For this review, take the finished solid that the model builds, in its own axes (mm). A direction names the side the tool comes from. Coordinates: 2 decimals unless noted, no trailing zeros. Write each loop counter-clockwise with the first axis right and the second up, starting at its lowest first coordinate (ties: lowest second). Pieces come first, ordered by that corner, then holes.
1) For faces 1 (the face through (6.583, 24.324, -1.479)), 2 (the face through (4.31, 17.88, -1.48)), list the 3-axis set-ups (+Z, -Z, +X, -X, +Y, -Y) from which the entire face can be reached by the end or side of a thin tool; tool diameter is ignored.
2) We need section C-C on y = -2.5. Write out the cut boundary in (x, z).
3) Insertion check: P1, Ø1, axis at y = 1, z = -1, coming from the +X side; P2, Ø1.5, axis at y = 2, z = -0.5, coming from the +X side; P3, Ø1.5, axis at x = 1, z = -1, coming from the -Y side. Each pin has a flat end and moves straight along its axis. Give the tip position at first contact, or say it passes through.
4) To check wall thickness, follow line 1 along X through (y, z) = (-4, -2.8); line 2 along Y through (x, z) = (-3.5, -1.55); line 3 along X through (y, z) = (-6, -0.1). State the ranges of each line that lie inside material, in increasing order.
5) Mouldability with a two-part tool opening along X and no side actions: class faces 3 (the face through (-4.88, -8.31, -1.48)), 4 (the face through (9.96, 10.462, -1.479)), 5 (the face through (-4.81, 5.69, -1.48)), 6 (the face through (0, 1, -3)) as pulls with the +X half, pulls with the -X half, needs draft (parallel to the pull), parting line crosses it, or undercut.
6) We need section B-B on z = -1.4. Write out the cut boundary in (x, y).
7) We need section A-A on y = 14. Write out the cut boundary in (x, z), then the cut area to 3 significant figures.
8) We need section D-D on y = -11. Write out the cut boundary in (x, z), then the cut area to 3 significant figures.
from build123d import *

# Parameters (mm, degrees)
F1_DEPTH = 3


with BuildPart() as f1:
    # F0 (on Top) → F1 (new body)
    with BuildSketch(Plane.XY):
        with BuildLine():
            Line((3.145587, 13.081894), (-1.617252, 14.912562))
            ThreePointArc((-1.617252, 14.912562), (-5.38163, -14.001359), (11.189027, 9.990279))
            Line((11.189027, 9.990279), (8.696999, 10.948126))
            ThreePointArc((8.696999, 10.948126), (10.035784, 16.738453), (9.370891, 22.644226))
            ThreePointArc((9.370891, 22.644226), (6.534897, 24.324435), (3.698903, 22.644226))
            ThreePointArc((3.698903, 22.644226), (4.30714, 17.811856), (3.145587, 13.081894))
        make_face()
        with BuildLine():
            ThreePointArc((5.58474, -8.803174), (-6.250082, -12.977674), (-8.510819, -0.633504))
            ThreePointArc((-8.510819, -0.633504), (-7.689946, -2.608119), (-6.533715, -4.407026))
            Line((-6.533715, -4.407026), (-8.664479, -8.012936))
            Line((-8.664479, -8.012936), (-5.728126, -9.748053))
            Line((-5.728126, -9.748053), (-4.006592, -6.834687))
            Line((-4.006592, -6.834687), (-2.219331, -7.890795))
            Line((-2.219331, -7.890795), (-3.654934, -10.320276))
            Line((-3.654934, -10.320276), (-1.297309, -11.713418))
            Line((-1.297309, -11.713418), (0.423625, -8.801069))
            ThreePointArc((0.423625, -8.801069), (3.004069, -9.081008), (5.58474, -8.803174))
        make_face(mode=Mode.SUBTRACT)
        Polygon((0.793802, -6.401524), (-4.951228, -3.248764), (0, -1.216984), align=None, mode=Mode.SUBTRACT)
        Polygon((8.780796, -3.59907), (3.386073, -0.866678), (9.691594, 4.73823), align=None, mode=Mode.SUBTRACT)
        Polygon((-3.222847, 1.18529), (-7.888624, 3.184909), (-1.639816, 8.267273), align=None, mode=Mode.SUBTRACT)
    extrude(amount=-F1_DEPTH)


solid = f1.part
Result:
1. face 1: +Z, -Z, +Y
1. face 2: +Z, -Z
2. outline: (-14.79, -3) - (-9.66, -3) - (-9.66, 0) - (-14.79, 0) - close; (-7.75, -3) - (-3.13, -3) - (-3.13, 0) - (-7.75, 0) - close; (0.2, -3) - (6.61, -3) - (6.61, 0) - (0.2, 0) - close; (8.9, -3) - (14.79, -3) - (14.79, 0) - (8.9, 0) - close
3. P1: stops at x = 14.99
3. P2: stops at x = 14.95
3. P3: stops at y = -15
4. line 1: x = -14.46 to -10.15, -6.84 to -3.58, 0.43 to 14.46
4. line 2: y = -14.59 to -13.97, -10.41 to -10.06, -7.13 to -4.05, -2.65 to 1.3, 6.75 to 14.59
4. line 3: x = -13.75 to -10.36, -7.48 to 0.06, 0.73 to 13.75
5. face 3: undercut
5. face 4: pulls with the +X half
5. face 5: undercut
5. face 6: needs draft
6. outline: (-1.62, 14.91) arc R15 ccw (long way) to (11.19, 9.99) - (8.7, 10.95) arc R17.6 ccw to (9.37, 22.64) arc R3.23 ccw to (3.7, 22.64) arc R13.38 cw to (3.15, 13.08) - close; hole (-8.66, -8.01) - (-6.53, -4.41) arc R12.08 cw to (-8.51, -0.63) arc R8.25 ccw (long way) to (5.58, -8.8) arc R12.08 cw to (0.42, -8.8) - (-1.3, -11.71) - (-3.65, -10.32) - (-2.22, -7.89) - (-4.01, -6.83) - (-5.73, -9.75) - close; hole (-7.89, 3.18) - (-3.22, 1.19) - (-1.64, 8.27) - close; hole (-4.95, -3.25) - (0.79, -6.4) - (0, -1.22) - close; hole (3.39, -0.87) - (8.78, -3.6) - (9.69, 4.74) - close
7. outline: (-5.39, -3) - (0.76, -3) - (0.76, 0) - (-5.39, 0) - close; (3.52, -3) - (9.66, -3) - (9.66, 0) - (3.52, 0) - close
7. area: 36.8 mm2
8. outline: (-10.2, -3) - (-8.55, -3) - (-8.55, 0) - (-10.2, 0) - close; (-2.5, -3) - (-0.88, -3) - (-0.88, 0) - (-2.5, 0) - close; (4.32, -3) - (10.2, -3) - (10.2, 0) - (4.32, 0) - close
8. area: 27.5 mm2
